```python
from build123d import *
from build123d.topology import SkipClean

# Parameters (mm, degrees)
SKETCH_3_W          = 6
SKETCH_3_H          = 70
SKETCH_2_R          = 4.4
CUT_EXTRUDE_1_DEPTH = 70
CUT_EXTRUDE_2_DEPTH = 10
FILLET_2_R          = 5
FILLET_3_DEPTH      = 4


with BuildPart() as part:
    # Эскиз1 → Повернуть2 (revolve)
    with BuildSketch(Plane.XY, mode=Mode.PRIVATE) as revolve_2_sk:
        with BuildLine():
            Line((0, 0), (49.6, 0))
            Line((49.6, 0), (49.6, 15))
            ThreePointArc((49.6, 15), (36.508962008, 96.668362047), (0.895786477, 171.319539959))
            ThreePointArc((0.895786477, 171.319539959), (0.493902777, 171.803280928), (0, 172.192608398))
            Line((0, 172.192608398), (0, 171.164859777))
            ThreePointArc((0, 171.164859777), (0.121207527, 171.025091653), (0.230243416, 170.875634074))
            ThreePointArc((0.230243416, 170.875634074), (35.74423335, 96.433414941), (48.8, 14.993655439))
            Line((48.8, 14.993655439), (48.8, 4))
            Line((48.8, 4), (0, 4))
            Line((0, 4), (0, 0))
        make_face()
    revolve(revolve_2_sk.sketch.rotate(Axis((0, 0, 0), (0, 1, 0)), 90), axis=Axis((0, 0, 0), (0, 1, 0)))

    # Эскиз3 → Повернуть6 (revolve)
    with BuildSketch(Plane.XY, mode=Mode.PRIVATE) as revolve_6_sk:
        with Locations((3, 39)):
            Rectangle(SKETCH_3_W, SKETCH_3_H)
    revolve(revolve_6_sk.sketch.rotate(Axis((0, 170.875634074, 0), (0, -1, 0)), 270), axis=Axis((0, 170.875634074, 0), (0, -1, 0)))

    # Эскиз2 → Вырез-Вытянуть1 (cut)
    with BuildSketch(Plane.XZ):
        with Locations(Location((0, 0, 0), (0, 0, 270))):
            Circle(SKETCH_2_R)
    extrude(amount=-CUT_EXTRUDE_1_DEPTH, mode=Mode.SUBTRACT)

    # Эскиз4 → Вырез-Вытянуть2 (cut)
    with BuildSketch(Plane.XZ):
        with BuildLine():
            ThreePointArc((48.543176657, 5), (34.506810922, 34.506810922), (5, 48.543176657))
            Line((5, 48.543176657), (5, 5))
            Line((5, 5), (48.543176657, 5))
        make_face()
        with BuildLine():
            Line((-5, 5), (-5, 48.543176657))
            ThreePointArc((-5, 48.543176657), (-34.506810922, 34.506810922), (-48.543176657, 5))
            Line((-48.543176657, 5), (-5, 5))
        make_face()
        with BuildLine():
            ThreePointArc((5, -48.543176657), (34.506810922, -34.506810922), (48.543176657, -5))
            Line((48.543176657, -5), (5, -5))
            Line((5, -5), (5, -48.543176657))
        make_face()
        with BuildLine():
            Line((-5, -5), (-48.543176657, -5))
            ThreePointArc((-48.543176657, -5), (-34.506810922, -34.506810922), (-5, -48.543176657))
            Line((-5, -48.543176657), (-5, -5))
        make_face()
    extrude(amount=-CUT_EXTRUDE_2_DEPTH, mode=Mode.SUBTRACT)

    # Скругление2
    # the kernel refuses this fillet: 5 mm, written as the material it adds along each edge
    with BuildSketch(Plane(origin=(48.543176657, 0, 5), x_dir=(-0.16572247027257606, 0, 0.9861724305854199), z_dir=(0, 1, 0)), Plane(origin=(5, 0, -48.543176657), x_dir=(0.9861724305854203, 0, 0.16572247027257497), z_dir=(0, 1, 0))) as fillet_2_piece_1:
        with BuildLine():
            CenterArc((5.908625729, -4.989810949), FILLET_2_R, 86.34158246, 103.197624337)
            Line((0.977763576, -5.818423301), (0, 0))
            ThreePointArc((0, 0), (3.113832998, 0.099445136), (6.227665995, 0))
        make_face()
    extrude(amount=4)
    with BuildSketch(Plane(origin=(5, 0, 48.543176657), x_dir=(0.9861724305854201, 0, -0.1657224702725758), z_dir=(0, 1, 0)), Plane(origin=(48.543176657, 0, -5), x_dir=(-0.16572247027257642, 0, -0.98617243058542), z_dir=(0, 1, 0))) as fillet_2_piece_2:
        with BuildLine():
            CenterArc((5.908625729, 4.989810949), FILLET_2_R, 170.460793203, 103.197624337)
            Line((0.977763576, 5.818423301), (0, 0))
            ThreePointArc((0, 0), (3.113832998, -0.099445136), (6.227665995, 0))
        make_face()
    extrude(amount=4)
    with BuildSketch(Plane(origin=(-48.543176657, 0, -5), x_dir=(1, 0, 0), z_dir=(0, 1, 0)), Plane(origin=(-5, 0, 48.543176657), x_dir=(0, 0, -1), z_dir=(0, 1, 0))) as fillet_2_piece_3:
        with BuildLine():
            CenterArc((5.900006044, 5), FILLET_2_R, 166.802375663, 103.197624337)
            ThreePointArc((1.032064193, 6.141552511), (0.417962045, 3.087256549), (0, 0))
            Line((0, 0), (5.900006044, 0))
        make_face()
    extrude(amount=4)
    with BuildSketch(Plane(origin=(-5, 0, -48.543176657), x_dir=(0, 0, 1), z_dir=(0, 1, 0)), Plane(origin=(-48.543176657, 0, 5), x_dir=(1, 0, 0), z_dir=(0, 1, 0))) as fillet_2_piece_4:
        with BuildLine():
            CenterArc((5.900006044, -5), FILLET_2_R, 90, 103.197624337)
            ThreePointArc((1.032064193, -6.141552511), (0.417962045, -3.087256549), (0, 0))
            Line((0, 0), (5.900006044, 0))
        make_face()
    extrude(amount=4)

    # Скругление3: read off the stored shape, not the designer's step
    # Скругление3 outline → Скругление3 (add)
    with SkipClean():  # the faces are left unmerged after this step: merging them gives an invalid solid
        with BuildSketch(Plane(origin=(0, 0, 0), x_dir=(1, 0, 0), z_dir=(0, 1, 0))):
            with BuildLine():
                Line((5, 5), (7, 5))
                ThreePointArc((7, 5), (5.585786438, 5.585786438), (5, 7))
                Line((5, 7), (5, 5))
            make_face()
            with BuildLine():
                Line((5, -5), (5, -7))
                ThreePointArc((5, -7), (5.585786438, -5.585786438), (7, -5))
                Line((7, -5), (5, -5))
            make_face()
            with BuildLine():
                Line((-5, 5), (-5, 7))
                ThreePointArc((-5, 7), (-5.585786438, 5.585786438), (-7, 5))
                Line((-7, 5), (-5, 5))
            make_face()
            with BuildLine():
                Line((-5, -5), (-7, -5))
                ThreePointArc((-7, -5), (-5.585786438, -5.585786438), (-5, -7))
                Line((-5, -7), (-5, -5))
            make_face()
        extrude(amount=FILLET_3_DEPTH)
    add(part.part.scale(1), mode=Mode.REPLACE)  # the faces are merged on a copy


solid = part.part
```
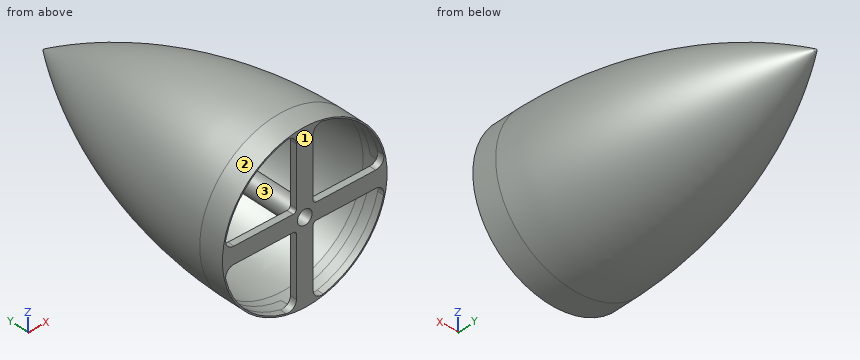
CAD build for the part. Positions are in the model's coordinates, mm. Face numbers are marked on the shaded views. Round coordinates to 2 decimals unless told otherwise and drop trailing zeros. Return JSON: item names as keys, results as strings. Group by question number.
Q1. Drill centre lines: line 1 along X through (y, z) = (10, 0); line 2 along X through (y, z) = (39, 0); line 3 along X through (y, z) = (78, -20). Where is each one in solid material? Low to high. Write a range as [from, to].
Q2. Two-plate mould, pull along Z, no slides. Class the marked faces 1, 2 and 3: +Z half, -Z half, draft (parallel to the pull), parting line (faces both ways), or undercut.
Q3. Flat gauge pins, fed straight in: pin 1 Ø4 at (y, z) = (57, -23) entering from +X; pin 2 Ø2 at (y, z) = (40, 2.5) entering from -X; pin 3 Ø4 at (x, y) = (-18.5, 86) entering from -Z; pin 4 Ø7 at (x, z) = (-1.5, 1.5) entering from -Y. Where does each tip first touch, or does it go through?
Q4. Band-saw the part on A-A on y = 30. Give the number of separate pieces and of enclosed holes in the cut face, plus the area to 3 significant figures.
Solutions:
{
 "1": {"line 1": "x = [-49.6, -48.8], [-6, -4.4], [4.4, 6], [48.8, 49.6]", "line 2": "x = [-48.22, -47.42], [-6, -4.4], [4.4, 6], [47.42, 48.22]", "line 3": "x = [-36.53, -35.59], [35.59, 36.53]"},
 "2": {"face 1": "draft", "face 2": "parting line", "face 3": "undercut"},
 "3": {"pin 1": "stops at x = 40.84", "pin 2": "stops at x = -48.17", "pin 3": "stops at z = -36.18", "pin 4": "stops at y = 0"},
 "4": {"separate pieces": "2", "enclosed holes": "2", "area": "297 mm^2"}
}
